Autodesk Fusion 360 part; units mm, degrees
sketch "スケッチ1" plane through (0, 0, 0) normal (0, 0, 1) x (1, 0, 0)
  circle A0 centre (0, 0) radius 10.5
  circle A1 centre (0, 0) radius 9.5
  circle A2 centre (0, 0) radius 9
  circle A3 centre (0, 0) radius 8
  dimension "d1" = 21
  dimension "d2" = 19
  dimension "d3" = 18
  dimension "d4" = 16
extrude "押し出し1" add sketch "スケッチ1" along normal blind 6 contours A0 makes body 1
extrude "押し出し2" add sketch "スケッチ1" along normal blind 6 separate body contours A2 makes body 2
sketch "スケッチ2" plane through (0, 0, 6) normal (0, 0, 1) x (-1, 0, 0)
  circle A0 centre (0, 0) radius 9.5
  circle A1 centre (0, 0) radius 10.5
  line L0 (2, -15) -> (-2, -15)
  line L1 (-2, -15) -> (-8.4577, -6.2223)
  line L2 (2, -15) -> (8.4577, -6.2223)
  line L3 (0, 0) -> (-3.4838, 0)
  line L4 (2, 15) -> (8.4577, 6.2223)
  line L5 (2, 15) -> (-2, 15)
  line L6 (-2, 15) -> (-8.4577, 6.2223)
extrude "押し出し3" add sketch "スケッチ2" against normal blind 2 contours A1 L4 L5 L6 | A1 L0 L1 L2 bodies 1
sketch "スケッチ3" plane through (0, 0, 6) normal (0, 0, 1) x (-1, 0, 0)
  circle A0 centre (0, 0) radius 8
  circle A1 centre (0, 0) radius 9
  line L0 (-15, -2) -> (-15, 2)
  line L1 (-15, 2) -> (-4.3494, 7.8792)
  line L2 (-15, 0) -> (-12.4057, 0)
  line L3 (-15, -2) -> (-4.3494, -7.8792)
  line L4 (0, 0) -> (0, -2)
  line L5 (15, -2) -> (4.3494, -7.8792)
  line L6 (15, -2) -> (15, 2)
  line L7 (15, 2) -> (4.3494, 7.8792)
extrude "押し出し4" add sketch "スケッチ3" along normal blind 2 separate body makes body 3
combine "結合1" operation add target body 3 tool bodies 2
sketch "スケッチ1 (2)" plane through (0, 0, 0) normal (0, 0, 1) x (1, 0, 0) in component "Component'"
  circle A0 centre (0, 0) radius 11.25
  circle A1 centre (0, 0) radius 9.75
  line L0 (-2.095, 15.0718) -> (2.1708, 15.0718)
  line L1 (2.1708, 15.0718) -> (8.6891, 7.1458)
  line L2 (-2.095, 15.0718) -> (-8.6482, 7.1952)
  line L3 (-5.0595, -20.013) -> (5.0595, -20.013)
  line L4 (5.0595, -20.013) -> (10.6475, -3.6322)
  line L5 (-5.0595, -20.013) -> (-10.6475, -3.6322)
  dimension "d13" = 22.5
  dimension "d14" = 19.5
extrude "押し出し1'" add sketch "スケッチ1 (2)" against normal blind 2 separate body makes body 4 in component "Component'"
extrude "押し出し2'" add sketch "スケッチ1 (2)" against normal blind 5 contours A0 bodies 4 in component "Component'"
sketch "スケッチ2 (2)" plane through (0, 0, 0) normal (0, 0, 1) x (1, 0, 0) in component "Component'"
  circle A0 centre (0, 0) radius 9
  circle A1 centre (0, 0) radius 8
  line L0 (14, 5) -> (14, -5)
  line L1 (14, -5) -> (2.722, -8.5785)
  line L2 (14, 5) -> (2.722, 8.5785)
  line L3 (0, 2) -> (0, 4)
  line L4 (-14, 5) -> (-14, -5)
  line L5 (-14, 5) -> (-2.722, 8.5785)
  line L6 (-14, -5) -> (-2.722, -8.5785)
  dimension "d19" = 18
  dimension "d20" = 16
extrude "押し出し3'" add sketch "スケッチ2 (2)" against normal blind 5 separate body contours A0 makes body 5 in component "Component'"
extrude "押し出し4'" add sketch "スケッチ2 (2)" against normal blind 2 contours A0 L0 L1 L2 | A0 L4 L5 L6 bodies 5 in component "Component'"
component "Component'" placed x (1, 0, 0) y (0, 1, 0) z (0, 0, 1) at (0, 0, 0)
hidden bodies 1 3 4
Read the model definition and answer for the solid it produces. Units are mm, in the model's axes. Give positions to 0.01 mm unless a question says otherwise; leave off trailing zeros. Loops run counter-clockwise (first coordinate to the right, second up) from the corner with the lowest first, then second, coordinate; pieces in that order, holes last. Notation, with made-up numbers: M 6.25,-25.75 L 21.25,-25.75 A26 cw 21.25,-2.75 Z; hole C -8,6.25 d1. An arc over 180 degrees is marked long. Write each question's results on one line, items separated by ' | '.
1. Section B-B on z = -1.25 is taken. Give the vertices of the cut face in (x, y).
Values:
outline: M -14,-5 L -2.72,-8.58 A9 ccw 2.72,-8.58 L 14,-5 L 14,5 L 2.72,8.58 A9 ccw -2.72,8.58 L -14,5 Z; hole C 0,0 d16
2. Section D-D on x = 7.5 is taken. Give the vertices of the cut face in (y, z), plus the area to 3 significant figures.
Values:
outline: M -7.06,-2 L -4.97,-2 L -4.97,-5 L -2.78,-5 L -2.78,0 L -7.06,0 Z; M 2.78,-5 L 4.97,-5 L 4.97,-2 L 7.06,-2 L 7.06,0 L 2.78,0 Z | area: 30.3 mm^2
3. Section C-C on y = 0 is taken. Give the vertices of the cut face in (x, z).
Values:
outline: M -14,-2 L -9,-2 L -9,-5 L -8,-5 L -8,0 L -14,0 Z; M 8,-5 L 9,-5 L 9,-2 L 14,-2 L 14,0 L 8,0 Z
4. Given pin 1 (1 mm diameter, centred on y = 0, z = -3, fed in from -X); pin 2 (2 mm diameter, centred on y = 1, z = -4.5, fed in from +X); pin 3 (1.5 mm diameter, centred on x = -11, z = -2, fed in from +Y), each flat-ended and moving along its own axis, determine where each tip first touches the part or whether it passes through.
Values:
pin 1: stops at x = -9 | pin 2: stops at x = 9 | pin 3: stops at y = 6.19
5. Straight lines are drawn through the part: line 1 (Y direction, x = 0, z = -3.65); line 2 (X direction, y = -4, z = -1.7); line 3 (Z direction, x = 11.75, y = 5.5). For each, find the intervals that lie inside material, in ascending order. Write a range as [from, to].
Values:
line 1: y = [-9, -8], [8, 9] | line 2: x = [-14, -6.93], [6.93, 14] | line 3: z = [-2, 0]
6. The mould has two halves that part along Y. Classify faces 1 (the face through (-1.73, -7.81, -2.46)), 2 (the face through (-9, 0, -3)), 3 (the face through (-8.44, 6.764, -0.986)), 4 (the face through (-11, 0, -2)): pulls with the +Y half, pulls with the -Y half, needs draft (parallel to the pull), parting line crosses it, or undercut.
Values:
face 1: undercut | face 2: parting line crosses it | face 3: pulls with the +Y half | face 4: needs draft
7. Section A-A on x = 0 is taken. Give the vertices of the cut face in (y, z), plus the area to 3 significant figures.
Values:
outline: M -9,-5 L -8,-5 L -8,0 L -9,0 Z; M 8,-5 L 9,-5 L 9,0 L 8,0 Z | area: 10.0 mm^2
